Verification items for the finished model (mm, model axes). Face numbers are marked on the shaded views. A direction names the side the tool comes from. Coordinates: 2 decimals unless noted, no trailing zeros. Write each loop counter-clockwise with the first axis right and the second up, starting at its lowest first coordinate (ties: lowest second). Pieces come first, ordered by that corner, then holes. Notation, with made-up numbers: (19, 47) -> (35, 47) arc R17 ccw to (35, 52) -> close; hole circle Ø1 at (-33.5, 33). An arc over 180 degrees is marked (long way). Write each question's results on one line, items separated by ' | '. Start each with the question number.
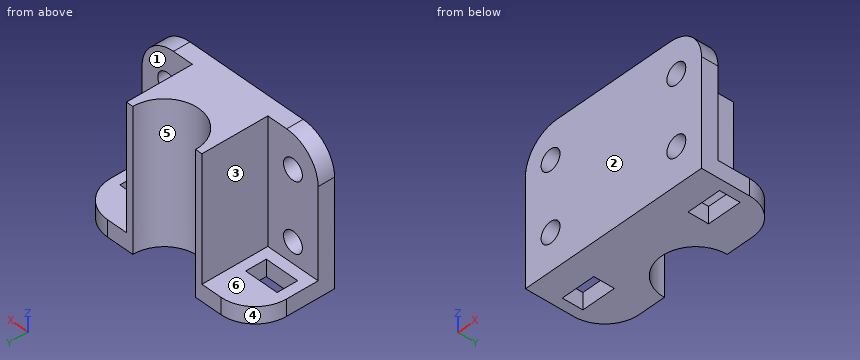
from build123d import *

# Parameters (mm, degrees)
BOSS_EXTRUDE1_DEPTH = 102
SKETCH2_W           = 40
SKETCH2_H           = 48
CUT_EXTRUDE1_DEPTH  = 90
FILLET1_R           = 25
FILLET2_R           = 25
SKETCH3_W           = 25
SKETCH3_H           = 15
CUT_EXTRUDE2_DEPTH  = 90
HOLE1_D             = 15


with BuildPart() as part:
    # Sketch1 → Boss-Extrude1 (new body)
    with BuildSketch(Plane.XY):
        with BuildLine():
            Line((-70, 0), (70, 0))
            Line((70, 0), (70, 60))
            Line((70, 60), (25, 60))
            ThreePointArc((25, 60), (0, 35), (-25, 60))
            Line((-25, 60), (-70, 60))
            Line((-70, 60), (-70, 0))
        make_face()
    extrude(amount=BOSS_EXTRUDE1_DEPTH)

    # Sketch2 → Cut-Extrude1 (cut)
    with BuildSketch(Plane.XY.offset(102)):
        with Locations((50, 36)):
            Rectangle(SKETCH2_W, SKETCH2_H)
    cut_extrude1 = extrude(amount=-CUT_EXTRUDE1_DEPTH, mode=Mode.SUBTRACT)

    # Mirror1: Cut-Extrude1 across plane
    add(cut_extrude1.mirror(Plane(origin=(0, 0, 0), x_dir=(0, 0, 1), z_dir=(1, 0, 0))), mode=Mode.SUBTRACT)

    # Fillet1
    fillet1_edges = [part.edges().sort_by_distance(p)[0] for p in [
        (70, 60, 6),
        (-70, 60, 6),
    ]]
    fillet(fillet1_edges, radius=FILLET1_R)

    # Fillet2
    fillet2_edges = [part.edges().sort_by_distance(p)[0] for p in [
        (70, 6, 102),
        (-70, 6, 102),
    ]]
    fillet(fillet2_edges, radius=FILLET2_R)

    # Sketch3 → Cut-Extrude2 (cut)
    with BuildSketch(Plane.XY.offset(12)):
        with Locations((50, 27.5)):
            Rectangle(SKETCH3_W, SKETCH3_H)
    cut_extrude2 = extrude(amount=-CUT_EXTRUDE2_DEPTH, mode=Mode.SUBTRACT)

    # Mirror2: Cut-Extrude2 across plane
    add(cut_extrude2.mirror(Plane(origin=(0, 0, 0), x_dir=(0, 0, 1), z_dir=(1, 0, 0))), mode=Mode.SUBTRACT)

    # Hole1 (through all)
    with Locations(Plane(origin=(0, 12, 0), x_dir=(1, 0, 0), z_dir=(0, 1, 0))):
        with Locations((50, -77), (50, -27), (-50, -27), (-50, -77)):
            Hole(HOLE1_D / 2)


solid = part.part
1. Sectioned sample at C-C on x = 50. Record the cut outline in (y, z), plus the area to 3 significant figures.
2. Sectioned sample at D-D on y = 39. Record the cut outline in (x, z), plus the area to 3 significant figures.
3. Material ranges on probe 1 along X at (y, z) = (3, 77); probe 2 along Z at (x, y) = (-50, 8.5); probe 3 along X at (y, z) = (3, 29), recorded low to high. Write a range as from..to.
4. Mould release check, pull along X, two halves, no side actions. Record for the marked faces 4, 5 and 6: +X half, -X half, draft (parallel to the pull), parting line (faces both ways), or undercut.
5. Tool access check on the marked faces 1, 2 and 3. Record the directions out of +Z, -Z, +X, -X, +Y, -Y that give a thin tool (end or side, any length) a straight path to the whole face; none if there is none.
6. Sectioned sample at B-B on z = 27. Record the cut outline in (x, y).
7. Sectioned sample at A-A on y = 23. Record the cut outline in (x, z).
8. Depth check by flat-ended pin: pin 1 Ø1.5 at (x, z) = (-20.5, 50.5) entering from +Y; pin 2 Ø3.5 at (x, z) = (-53, 3.5) entering from -Y; pin 3 Ø13 at (x, z) = (-54.5, 8.5) entering from +Y; pin 4 Ø20 at (x, y) = (-40.5, 25) entering from +Z. Enter the tip coordinate at first touch or a pass-through.
Computed values:
1) outline: (0, 0) -> (20, 0) -> (20, 12) -> (12, 12) -> (12, 19.5) -> (0, 19.5) -> close; (0, 34.5) -> (12, 34.5) -> (12, 69.5) -> (0, 69.5) -> close; (0, 84.5) -> (12, 84.5) -> (12, 101.49) -> (0, 101.49) -> close; (35, 0) -> (59.49, 0) -> (59.49, 12) -> (35, 12) -> close | area: 1,250 mm^2
2) outline: (-69.68, 0) -> (-13.56, 0) -> (-13.56, 102) -> (-30, 102) -> (-30, 12) -> (-69.68, 12) -> close; (13.56, 0) -> (69.68, 0) -> (69.68, 12) -> (30, 12) -> (30, 102) -> (13.56, 102) -> close | area: 4,310 mm^2
3) probe 1: x = -70..-57.5, -42.5..42.5, 57.5..70 | probe 2: z = 0..19.5, 34.5..69.5, 84.5..101.49 | probe 3: x = -70..-57.23, -42.77..42.77, 57.23..70
4) face 4: -X half | face 5: undercut | face 6: draft
5) face 1: +Z, +X, +Y | face 2: +Z, -Z, +X, -X, -Y | face 3: +Z, -X, +Y
6) outline: (-70, 0) -> (-57.5, 0) -> (-57.5, 12) -> (-70, 12) -> close; (-42.5, 0) -> (42.5, 0) -> (42.5, 12) -> (30, 12) -> (30, 60) -> (25, 60) arc R25 cw to (-25, 60) -> (-30, 60) -> (-30, 12) -> (-42.5, 12) -> close; (57.5, 0) -> (70, 0) -> (70, 12) -> (57.5, 12) -> close
7) outline: (-70, 0) -> (-62.5, 0) -> (-62.5, 12) -> (-70, 12) -> close; (-37.5, 0) -> (37.5, 0) -> (37.5, 12) -> (30, 12) -> (30, 102) -> (-30, 102) -> (-30, 12) -> (-37.5, 12) -> close; (62.5, 0) -> (70, 0) -> (70, 12) -> (62.5, 12) -> close
8) pin 1: stops at y = 46.83 | pin 2: stops at y = 0 | pin 3: stops at y = 59.82 | pin 4: stops at z = 12
